```python
from build123d import *

# Parameters (mm, degrees)
PAD_DEPTH       = 71.2
POCKET_DEPTH    = 5.7
SKETCH001_R     = 4.2
SKETCH001_W     = 14.4
SKETCH001_H     = 30.4
POCKET001_DEPTH = 7.5
SKETCH003_W     = 41.7
SKETCH003_H     = 29
PAD001002_DEPTH = 2
POCKET002_DEPTH = 2
SKETCH005_W     = 2.9
SKETCH005_H     = 10.8
POCKET003_DEPTH = 4
SKETCH006_W     = 8.8
SKETCH006_H     = 14.2
POCKET004_DEPTH = 7.201
FILLET_R        = 6


with BuildPart() as part:
    # Sketch → Pad (new body)
    with BuildSketch(Plane.YZ):
        Polygon((0, 0), (0, 58), (29.698485, 87.698485), (34.789654, 82.607316), (7.2, 55.017662), (7.2, 29), (41.7, 29), (41.7, 26), (12.7, 26), (12.7, 3), (41.7, 3), (41.7, 0), align=None)
    extrude(amount=PAD_DEPTH)

    # Sketch002 (on Face8 of Pad) → Pocket (cut)
    with BuildSketch(Plane(origin=(0, -23.908831, 23.908831), x_dir=(0, 0.707107, 0.707107), z_dir=(0, 0.707107, -0.707107))):
        Polygon((56.394531, 50.3), (56.394531, 37.9), (53.394531, 37.9), (53.394531, 37), (51.994531, 37), (51.994531, 37.9), (48.394531, 37.9), (48.394531, 37), (46.994531, 37), (46.994531, 37.9), (43.994531, 37.9), (43.994531, 50.3), (46.994531, 50.3), (46.994531, 51.2), (48.394531, 51.2), (48.394531, 50.3), (51.994531, 50.3), (51.994531, 51.2), (53.394531, 51.2), (53.394531, 50.3), align=None)
        Polygon((43.994531, 20.9), (46.994531, 20.9), (46.994531, 20), (48.394531, 20), (48.394531, 20.9), (51.994531, 20.9), (51.994531, 20), (53.394531, 20), (53.394531, 20.9), (56.394531, 20.9), (56.394531, 33.3), (53.394531, 33.3), (53.394531, 34.2), (51.994531, 34.2), (51.994531, 33.3), (48.394531, 33.3), (48.394531, 34.2), (46.994531, 34.2), (46.994531, 33.3), (43.994531, 33.3), align=None)
    extrude(amount=-POCKET_DEPTH, mode=Mode.SUBTRACT)

    # Sketch001 (on Face10 of Pocket) → Pocket001 (cut)
    with BuildSketch(Plane(origin=(0, -29, 29), x_dir=(0, -0.707107, -0.707107), z_dir=(0, -0.707107, 0.707107))):
        with Locations((-50.195, 44.1)):
            Circle(SKETCH001_R)
        with Locations((-50.195, 27.1)):
            Circle(SKETCH001_R)
        with Locations((-67.995, 35.6)):
            Rectangle(SKETCH001_W, SKETCH001_H)
    extrude(amount=-POCKET001_DEPTH, mode=Mode.SUBTRACT)

    # Sketch003 (on Face5 of Pocket001) → Pad001002 (join)
    with BuildSketch(Plane.YZ.offset(71.2)):
        with Locations((20.85, 14.5)):
            Rectangle(SKETCH003_W, SKETCH003_H)
    extrude(amount=-PAD001002_DEPTH)

    # Sketch004 (on Face8 of Pad001002) → Pocket002 (cut)
    with BuildSketch(Plane(origin=(0, -23.908831, 23.908831), x_dir=(0, 0.707107, 0.707107), z_dir=(0, 0.707107, -0.707107))):
        with BuildLine():
            ThreePointArc((64.247016, 55.7), (63.347016, 54.8), (64.247016, 53.9))
            Line((64.247016, 53.9), (71.867016, 53.9))
            ThreePointArc((71.867016, 53.9), (72.767016, 54.8), (71.867016, 55.7))
            Line((64.247016, 55.7), (71.867016, 55.7))
        make_face()
        with BuildLine():
            ThreePointArc((64.247016, 13.3), (63.347016, 12.4), (64.247016, 11.5))
            Line((64.247016, 11.5), (71.867016, 11.5))
            ThreePointArc((71.867016, 11.5), (72.767016, 12.4), (71.867016, 13.3))
            Line((64.247016, 13.3), (71.867016, 13.3))
        make_face()
    extrude(amount=-POCKET002_DEPTH, mode=Mode.SUBTRACT)

    # Sketch005 (on Face13 of Pocket002) → Pocket003 (cut)
    with BuildSketch(Plane(origin=(0, 0, 29), x_dir=(0, -1, 0), z_dir=(0, 0, 1))):
        with Locations((-14.15, 60.2)):
            Rectangle(SKETCH005_W, SKETCH005_H)
    extrude(amount=-POCKET003_DEPTH, mode=Mode.SUBTRACT)

    # Sketch006 (on Face11 of Pocket003) → Pocket004 (cut, through all)
    with BuildSketch(Plane.ZX.offset(7.2)):
        with Locations((33.4, 54.6)):
            Rectangle(SKETCH006_W, SKETCH006_H)
    extrude(amount=-POCKET004_DEPTH, mode=Mode.SUBTRACT)

    # Fillet
    fillet_edges = [part.edges().sort_by_distance(p)[0] for p in [
        (71.2, 32.244069, 85.1529),
        (0, 32.244069, 85.1529),
    ]]
    fillet(fillet_edges, radius=FILLET_R)


solid = part.part
```
Source: CAD feature listing. Evaluate the final solid. Frame: model axes, mm. A direction names the side the tool comes from. Round coordinates to 2 decimals unless told otherwise and drop trailing zeros. Order: outer loops, then holes, each group sorted by start corner. A loop starts at its lowest first (then second) coordinate and runs counter-clockwise, first axis right, second up. Notation, with made-up numbers: (57, 32) -> (88, 32) arc R16 cw to (88, 42) -> close; hole circle Ø8 at (65.25, -13.5). An arc over 180 degrees is marked (long way). Use CSV: the item, a comma, the result in double quotes.
(1) Section D-D on y = 38. Return the cut outline in (x, z), and give its area (3 significant figures).
Report:
outline,"(0, 0) -> (71.2, 0) -> (71.2, 29) -> (0, 29) -> (0, 26) -> (69.2, 26) -> (69.2, 3) -> (0, 3) -> close"
area,"473 mm^2"
(2) First-contact query: pin 1 Ø6 at (x, y) = (54.5, 7) entering from +Z; pin 2 Ø2 at (y, z) = (23.5, 73.5) entering from -X; pin 3 Ø1 at (x, z) = (20, 12) entering from +Y. Flat tips, straight axial feed; report the tip coordinate or a pass-through.
Report:
pin 1,"z = 68"
pin 2,"x = 0"
pin 3,"y = 12.7"
(3) Access query for faces 4 (the face through (54.82, 20.187, 69.399)), 5 (the face through (33.76, 10.87, 62.66)), 6 (the face through (47.5, 4, 33)). Directions: +Z, -Z, +X, -X, +Y, -Y. A direction counts if a zero-diameter tool reaches every point of the face in a straight line with its end or side. Return the directions, or none.
Report:
face 4,"+Y"
face 5,"none"
face 6,"+Y, -Y"
(4) Section C-C on x = 30. Return the cut outline in (y, z).
Report:
outline,"(0, 0) -> (41.7, 0) -> (41.7, 3) -> (12.7, 3) -> (12.7, 26) -> (41.7, 26) -> (41.7, 29) -> (7.2, 29) -> (7.2, 55.02) -> (3.17, 59.05) -> (5.41, 61.28) -> (4.34, 62.34) -> (0, 58) -> close; (8.64, 66.64) -> (9.7, 65.58) -> (11.94, 67.82) -> (15.97, 63.79) -> (19.08, 66.9) -> (13.99, 71.99) -> close; (24.17, 82.17) -> (29.26, 77.08) -> (34.79, 82.61) -> (29.7, 87.7) -> close"
(5) Section B-B on y = 18. Return the cut outline in (x, z).
Report:
outline,"(0, 0) -> (71.2, 0) -> (71.2, 29) -> (0, 29) -> (0, 26) -> (69.2, 26) -> (69.2, 3) -> (0, 3) -> close; (0, 65.82) -> (71.2, 65.82) -> (71.2, 76) -> (50.8, 76) -> (50.8, 67.98) -> (20.4, 67.98) -> (20.4, 76) -> (0, 76) -> close"
(6) Section A-A on x = 52.5. Return the cut outline in (y, z), and give its area (3 significant figures).
Report:
outline,"(0, 0) -> (41.7, 0) -> (41.7, 3) -> (12.7, 3) -> (12.7, 26) -> (41.7, 26) -> (41.7, 29) -> (0, 29) -> close; (0, 37.8) -> (7.2, 37.8) -> (7.2, 55.02) -> (34.79, 82.61) -> (29.7, 87.7) -> (0, 58) -> close"
area,"969 mm^2"
(7) Pull-direction query (Z, two-part tool) for faces 1 (the face through (0, 7, 36)), 2 (the face through (35, 21, 0)), 3 (the face through (33.74, 11.86, 63.65)); classes: +Z half, -Z half, draft (parallel to the pull), parting line (faces both ways), or undercut.
Report:
face 1,"draft"
face 2,"-Z half"
face 3,"undercut"
(8) Ray query, L1, parallel to Z at x = 57.5, y = 39; L2, parallel to Z at x = 27, y = 13.5; L3, parallel to Z at x = 12.5, y = 17. Return the intervals inside material, ascending.
Report:
L1,"0 to 3, 26 to 29"
L2,"0 to 3, 26 to 29, 66.25 to 71.5"
L3,"0 to 3, 26 to 29, 64.82 to 75"
